Read the model definition and answer for the solid it produces. Units are mm, in the model's axes. Face numbers are marked on the shaded views. Coordinates: 2 decimals unless noted, no trailing zeros. Write each loop counter-clockwise with the first axis right and the second up, starting at its lowest first coordinate (ties: lowest second). Pieces come first, ordered by that corner, then holes. Notation, with made-up numbers: M 6,-9.5 L 14,-9.5 A25 ccw 14,29.5 Z; hole C -4,-26 d9. An arc over 180 degrees is marked long. Write item = value, one per line.
from build123d import *

# Parameters (mm, degrees)
SKETCH1_R           = 3
SKETCH1_R_2         = 1.625
BOSS_EXTRUDE1_DEPTH = 6
FILLET1_R           = 0.25


with BuildPart() as part:
    # Sketch1 → Boss-Extrude1 (new body)
    with BuildSketch(Plane(origin=(0, 0, 0), x_dir=(1, 0, 0), z_dir=(0, 1, 0))):
        with Locations(Location((0, 0, 0), (0, 0, 270))):  # turned: the seam where the file's is
            Circle(SKETCH1_R)
        with Locations(Location((0, 0, 0), (0, 0, 270))):  # turned: the seam where the file's is
            Circle(SKETCH1_R_2, mode=Mode.SUBTRACT)
    extrude(amount=BOSS_EXTRUDE1_DEPTH)

    # Fillet1
    fillet1_edges = [part.edges().sort_by_distance(p)[0] for p in [
        (0, 0, -3),
        (0, 6, -3),
        (0, 0, -1.625),
        (0, 6, -1.625),
    ]]
    fillet(fillet1_edges, radius=FILLET1_R)


solid = part.part
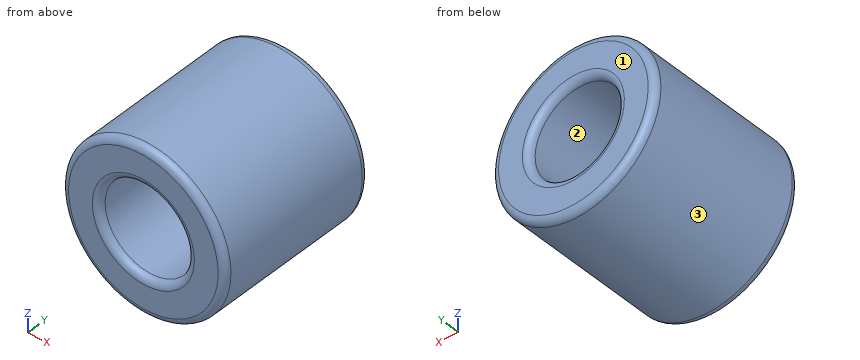
Item 1: Flat-ended cylindrical pins translate along their axes: pin 1 (2 mm diameter, centred on x = 1, y = 4.5, fed in from -Z); pin 2 (1.5 mm diameter, centred on x = 2, y = 3, fed in from +Z). Find the tip coordinate at first contact, or state that the pin passes through.
Worked answers:
pin_1 = -3
pin_2 = 2.73
Item 2: Consider line 1 along X through (y, z) = (3.3, 0) (3 decimals); line 2 along X through (y, z) = (4, 1). Determine where each line is inside the solid, lowest interval first. Write a range as from..to.
Worked answers:
line_1 = -3..-1.625, 1.625..3
line_2 = -2.83..-1.28, 1.28..2.83
Item 3: Find section A-A (x = 0). Determine the outline of the cut face in (y, z) (3 decimals), and give its area (3 significant figures).
Worked answers:
outline = M 0,-2.75 A0.25 ccw 0.25,-3 L 5.75,-3 A0.25 ccw 6,-2.75 L 6,-1.875 A0.25 ccw 5.75,-1.625 L 0.25,-1.625 A0.25 ccw 0,-1.875 Z; M 0,1.875 A0.25 ccw 0.25,1.625 L 5.75,1.625 A0.25 ccw 6,1.875 L 6,2.75 A0.25 ccw 5.75,3 L 0.25,3 A0.25 ccw 0,2.75 Z
area = 16.4 mm²
Item 4: Find section C-C (y = 2). Determine the outline of the cut face in (x, z) (3 decimals), and give its area (3 significant figures).
Worked answers:
outline = C 0,0 d6; hole C 0,0 d3.25
area = 20.0 mm²
Item 5: Find section B-B (z = 0). Determine the outline of the cut face in (x, y) (3 decimals).
Worked answers:
outline = M -3,0.25 A0.25 ccw -2.75,0 L -1.875,0 A0.25 ccw -1.625,0.25 L -1.625,5.75 A0.25 ccw -1.875,6 L -2.75,6 A0.25 ccw -3,5.75 Z; M 1.625,0.25 A0.25 ccw 1.875,0 L 2.75,0 A0.25 ccw 3,0.25 L 3,5.75 A0.25 ccw 2.75,6 L 1.875,6 A0.25 ccw 1.625,5.75 Z
Item 6: For a pull along Z with two mould halves and no side action, classify the marked faces 1, 2 and 3 as released by +Z, released by -Z, zero draft, split by the parting line, or undercut.
Worked answers:
face_1 = zero draft
face_2 = undercut
face_3 = split by the parting line
